```python
from build123d import *

# Parameters (mm, degrees)
SZKIC1_R                    = 4
SZKIC1_R_2                  = 1.5
DODANIE_WYCI_GNI_CIE1_DEPTH = 2
SZKIC2_R                    = 2.5
SZKIC2_R_2                  = 1.5
DODANIE_WYCI_GNI_CIE2_DEPTH = 4
SFAZOWANIE1_SIZE            = 1
SFAZOWANIE1_SIZE2           = 1.732050808


with BuildPart() as part:
    # Szkic1 → Dodanie-wyciągnięcie1 (new body)
    with BuildSketch(Plane(origin=(0, 0, 0), x_dir=(1, 0, 0), z_dir=(0, 1, 0))):
        with Locations(Location((0, 0, 0), (0, 0, 270))):
            Circle(SZKIC1_R)
        with Locations(Location((0, 0, 0), (0, 0, 270))):
            Circle(SZKIC1_R_2, mode=Mode.SUBTRACT)
    extrude(amount=DODANIE_WYCI_GNI_CIE1_DEPTH)

    # Szkic2 → Dodanie-wyciągnięcie2 (add)
    with BuildSketch(Plane(origin=(0, 2, 0), x_dir=(1, 0, 0), z_dir=(0, 1, 0))):
        with Locations(Location((0, 0, 0), (0, 0, 270))):
            Circle(SZKIC2_R)
        with Locations(Location((0, 0, 0), (0, 0, 270))):
            Circle(SZKIC2_R_2, mode=Mode.SUBTRACT)
    extrude(amount=DODANIE_WYCI_GNI_CIE2_DEPTH)

    # Sfazowanie1
    sfazowanie1_edges = [part.edges().sort_by_distance(p)[0] for p in [
        (0, 0, -4),
    ]]
    sfazowanie1_side = [part.faces().sort_by_distance(p)[0] for p in [
        (0, 1, -4),
    ]]
    chamfer(sfazowanie1_edges, length=SFAZOWANIE1_SIZE, length2=SFAZOWANIE1_SIZE2, reference=sfazowanie1_side[0])


solid = part.part
```
The model under review builds one solid part; all positions refer to its coordinate system, in mm. Round coordinates to 2 decimals unless told otherwise and drop trailing zeros. Loops run counter-clockwise (first coordinate to the right, second up) from the corner with the lowest first, then second, coordinate; pieces in that order, holes last. Notation, with made-up numbers: (50, 33.25) -> (102, 33.25) arc R17 ccw to (102, 61.25) -> close; hole circle Ø9 at (38.5, 43). An arc over 180 degrees is marked (long way). Answer as a JSON object with one key per item and string values. Group by question number.
1) We need section A-A on x = 0. Write out the cut boundary in (y, z), then the cut area to 3 significant figures.
2) We need section B-B on z = 0. Write out the cut boundary in (x, y), then the cut area to 3 significant figures.
3) For line 1 (X direction, y = 4.3, z = 0); line 2 (Z direction, x = -0.5, y = 4.9); line 3 (Z direction, x = 0.25, y = 4.05), list the stretches that pass through material, from the lowest coordinate up. Write a range as [from, to].
4) We need section D-D on y = 2.7. Write out the cut boundary in (x, z), then the cut area to 3 significant figures.
5) Mouldability with a two-part tool opening along X and no side actions: class faces 1 (the face through (-2.44, 3.97, -0.54)), 2 (the face through (0.45, 2.96, 1.43)), 3 (the face through (2, 2, 2)) as released by +X, released by -X, zero draft, split by the parting line, or undercut.
6) We need section C-C on y = 1.65. Write out the cut boundary in (x, z).
7) For pin 1 Ø2 at (x, z) = (-0.5, -1) entering from +Y; pin 2 Ø2 at (x, y) = (-2, 2.5) entering from +Z, all flat-tipped, find the tip position at first contact; note any pin that passes through.
Result set:
{
 "1": {"outline": "(0, -2.27) -> (1, -4) -> (2, -4) -> (2, -2.5) -> (6, -2.5) -> (6, -1.5) -> (0, -1.5) -> close; (0, 1.5) -> (6, 1.5) -> (6, 2.5) -> (2, 2.5) -> (2, 4) -> (1, 4) -> (0, 2.27) -> close", "area": "16.3 mm²"},
 "2": {"outline": "(-4, 1) -> (-2.27, 0) -> (-1.5, 0) -> (-1.5, 6) -> (-2.5, 6) -> (-2.5, 2) -> (-4, 2) -> close; (1.5, 0) -> (2.27, 0) -> (4, 1) -> (4, 2) -> (2.5, 2) -> (2.5, 6) -> (1.5, 6) -> close", "area": "16.3 mm²"},
 "3": {"line 1": "[-2.5, -1.5], [1.5, 2.5]", "line 2": "[-2.45, -1.41], [1.41, 2.45]", "line 3": "[-2.49, -1.48], [1.48, 2.49]"},
 "4": {"outline": "circle Ø5 at (0, 0); hole circle Ø3 at (0, 0)", "area": "12.6 mm²"},
 "5": {"face 1": "split by the parting line", "face 2": "undercut", "face 3": "zero draft"},
 "6": {"outline": "circle Ø8 at (0, 0); hole circle Ø3 at (0, 0)"},
 "7": {"pin 1": "y = 6", "pin 2": "z = 3.84"}
}
